Check sheet for the modelled part. Datum: model origin and axes. Units: mm. A direction names the side the tool comes from. Round coordinates to 2 decimals unless told otherwise and drop trailing zeros. Write each loop counter-clockwise with the first axis right and the second up, starting at its lowest first coordinate (ties: lowest second). Pieces come first, ordered by that corner, then holes. Notation, with made-up numbers: (-8.75, -2.75) -> (47.25, -2.75) arc R21 ccw to (47.25, 14.25) -> close; hole circle Ø11 at (-6, 23.25). An arc over 180 degrees is marked (long way). Put each result on its own line as item: value. Start each with the question number.
from build123d import *

# Parameters (mm, degrees)
SKETCH1_W              = 273.05
SKETCH1_H              = 139.7
BOSS_EXTRUDE1_DEPTH    = 5.588
SKETCH2_W              = 273.05
SKETCH2_H              = 139.7
SKETCH2_W_2            = 261.874
SKETCH2_H_2            = 128.524
BOSS_EXTRUDE2_DEPTH    = 298.45
SKETCH3_W              = 6.35
SKETCH3_H              = 16.933333333
SKETCH3_H_2            = 16.933333334
DOOR_SLOT_DEPTH        = 12.7
DOOR_GUIDE_HOLES_REACH = 361.255
SKETCH4_W              = 6.35
SKETCH4_H              = 15.875
LEVER_HOLES_W          = 9.652
LEVER_HOLES_H          = 6.35
LEVER_HOLES_W_2        = 6.35
CUT_EXTRUDE1_DEPTH     = 362.378293578
CUT_EXTRUDE3_REACH     = 416.577
SKETCH8_R              = 3.175
SKETCH16_W             = 327.238778096
SKETCH16_H             = 314.471565403
CUT_EXTRUDE10_DEPTH    = 362.378293578
LEFT_RIGHT_W           = 6.35
LEFT_RIGHT_H           = 5.588
LEFT_RIGHT_W_2         = 12.7
LEFT_RIGHT_H_2         = 12.66825
CUT_EXTRUDE11_DEPTH    = 415.577411883
SKETCH17_R             = 1.5
SKETCH17_W             = 23
SKETCH17_H             = 17.61800007
CUT_EXTRUDE12_DEPTH    = 313.00857951
CUT_EXTRUDE13_DEPTH    = 313.00857951


with BuildPart() as part:
    # Sketch1 → Boss-Extrude1 (new body)
    with BuildSketch(Plane(origin=(0, 0, 0), x_dir=(1, 0, 0), z_dir=(0, 1, 0))):
        Rectangle(SKETCH1_W, SKETCH1_H)
    extrude(amount=BOSS_EXTRUDE1_DEPTH)

    # Sketch2 → Boss-Extrude2 (add)
    with BuildSketch(Plane(origin=(0, 5.588, 0), x_dir=(1, 0, 0), z_dir=(0, 1, 0))):
        Rectangle(SKETCH2_W, SKETCH2_H)
        Rectangle(SKETCH2_W_2, SKETCH2_H_2, mode=Mode.SUBTRACT)
    extrude(amount=BOSS_EXTRUDE2_DEPTH)

    # Sketch3 → Door Slot (cut)
    with BuildSketch(Plane.XY.offset(69.85)):
        with BuildLine():
            Line((-29.337, 282.448), (-29.337, 5.588))
            Line((-29.337, 5.588), (-22.733, 5.588))
            Line((-22.733, 5.588), (-22.733, 291.592))
            Line((-22.733, 291.592), (-42.291, 291.592))
            Line((-42.291, 291.592), (-42.291, 284.988))
            Line((-42.291, 284.988), (-31.877, 284.988))
            ThreePointArc((-31.877, 284.988), (-30.080948776, 284.244051224), (-29.337, 282.448))
        make_face()
        with Locations((-13.208, 80.433333334)):
            Rectangle(SKETCH3_W, SKETCH3_H)
        with Locations((-13.208, 50.8)):
            Rectangle(SKETCH3_W, SKETCH3_H_2)
        with Locations((-13.208, 21.166666667)):
            Rectangle(SKETCH3_W, SKETCH3_H)
    extrude(amount=-DOOR_SLOT_DEPTH, mode=Mode.SUBTRACT)

    # Sketch4 → Door Guide Holes (cut, up to next)
    with BuildSketch(Plane.XY.offset(-64.262), mode=Mode.PRIVATE) as door_guide_holes_sk1:
        with Locations((-45.466, 283.4005)):
            Rectangle(SKETCH4_W, SKETCH4_H)
    door_guide_holes_tool1 = extrude(door_guide_holes_sk1.sketch, amount=-DOOR_GUIDE_HOLES_REACH, mode=Mode.PRIVATE) & part.part
    # Sketch4 → Door Guide Holes (cut, up to next)
    with BuildSketch(Plane.XY.offset(-64.262), mode=Mode.PRIVATE) as door_guide_holes_sk2:
        with Locations((-45.466, 254.8255)):
            Rectangle(SKETCH4_W, SKETCH4_H)
    door_guide_holes_tool2 = extrude(door_guide_holes_sk2.sketch, amount=-DOOR_GUIDE_HOLES_REACH, mode=Mode.PRIVATE) & part.part
    # Sketch4 → Door Guide Holes (cut, up to next)
    with BuildSketch(Plane.XY.offset(-64.262), mode=Mode.PRIVATE) as door_guide_holes_sk3:
        with Locations((-45.466, 226.2505)):
            Rectangle(SKETCH4_W, SKETCH4_H)
    door_guide_holes_tool3 = extrude(door_guide_holes_sk3.sketch, amount=-DOOR_GUIDE_HOLES_REACH, mode=Mode.PRIVATE) & part.part
    # Sketch4 → Door Guide Holes (cut, up to next)
    with BuildSketch(Plane.XY.offset(-64.262), mode=Mode.PRIVATE) as door_guide_holes_sk4:
        with Locations((-45.466, 197.6755)):
            Rectangle(SKETCH4_W, SKETCH4_H)
    door_guide_holes_tool4 = extrude(door_guide_holes_sk4.sketch, amount=-DOOR_GUIDE_HOLES_REACH, mode=Mode.PRIVATE) & part.part
    # Sketch4 → Door Guide Holes (cut, up to next)
    with BuildSketch(Plane.XY.offset(-64.262), mode=Mode.PRIVATE) as door_guide_holes_sk5:
        with Locations((-45.466, 169.1005)):
            Rectangle(SKETCH4_W, SKETCH4_H)
    door_guide_holes_tool5 = extrude(door_guide_holes_sk5.sketch, amount=-DOOR_GUIDE_HOLES_REACH, mode=Mode.PRIVATE) & part.part
    # Sketch4 → Door Guide Holes (cut, up to next)
    with BuildSketch(Plane.XY.offset(-64.262), mode=Mode.PRIVATE) as door_guide_holes_sk6:
        with Locations((-45.466, 140.5255)):
            Rectangle(SKETCH4_W, SKETCH4_H)
    door_guide_holes_tool6 = extrude(door_guide_holes_sk6.sketch, amount=-DOOR_GUIDE_HOLES_REACH, mode=Mode.PRIVATE) & part.part
    # Sketch4 → Door Guide Holes (cut, up to next)
    with BuildSketch(Plane.XY.offset(-64.262), mode=Mode.PRIVATE) as door_guide_holes_sk7:
        with Locations((-45.466, 111.9505)):
            Rectangle(SKETCH4_W, SKETCH4_H)
    door_guide_holes_tool7 = extrude(door_guide_holes_sk7.sketch, amount=-DOOR_GUIDE_HOLES_REACH, mode=Mode.PRIVATE) & part.part
    # Sketch4 → Door Guide Holes (cut, up to next)
    with BuildSketch(Plane.XY.offset(-64.262), mode=Mode.PRIVATE) as door_guide_holes_sk8:
        with Locations((-45.466, 83.3755)):
            Rectangle(SKETCH4_W, SKETCH4_H)
    door_guide_holes_tool8 = extrude(door_guide_holes_sk8.sketch, amount=-DOOR_GUIDE_HOLES_REACH, mode=Mode.PRIVATE) & part.part
    # Sketch4 → Door Guide Holes (cut, up to next)
    with BuildSketch(Plane.XY.offset(-64.262), mode=Mode.PRIVATE) as door_guide_holes_sk9:
        with Locations((-45.466, 54.8005)):
            Rectangle(SKETCH4_W, SKETCH4_H)
    door_guide_holes_tool9 = extrude(door_guide_holes_sk9.sketch, amount=-DOOR_GUIDE_HOLES_REACH, mode=Mode.PRIVATE) & part.part
    # Sketch4 → Door Guide Holes (cut, up to next)
    with BuildSketch(Plane.XY.offset(-64.262), mode=Mode.PRIVATE) as door_guide_holes_sk10:
        with Locations((-45.466, 26.2255)):
            Rectangle(SKETCH4_W, SKETCH4_H)
    door_guide_holes_tool10 = extrude(door_guide_holes_sk10.sketch, amount=-DOOR_GUIDE_HOLES_REACH, mode=Mode.PRIVATE) & part.part
    door_guide_holes_1 = door_guide_holes_tool1.solids().sort_by_distance((-45.466, 283.4005, -64.262))[0]
    add(door_guide_holes_1, mode=Mode.SUBTRACT)
    door_guide_holes_2 = door_guide_holes_tool2.solids().sort_by_distance((-45.466, 254.8255, -64.262))[0]
    add(door_guide_holes_2, mode=Mode.SUBTRACT)
    door_guide_holes_3 = door_guide_holes_tool3.solids().sort_by_distance((-45.466, 226.2505, -64.262))[0]
    add(door_guide_holes_3, mode=Mode.SUBTRACT)
    door_guide_holes_4 = door_guide_holes_tool4.solids().sort_by_distance((-45.466, 197.6755, -64.262))[0]
    add(door_guide_holes_4, mode=Mode.SUBTRACT)
    door_guide_holes_5 = door_guide_holes_tool5.solids().sort_by_distance((-45.466, 169.1005, -64.262))[0]
    add(door_guide_holes_5, mode=Mode.SUBTRACT)
    door_guide_holes_6 = door_guide_holes_tool6.solids().sort_by_distance((-45.466, 140.5255, -64.262))[0]
    add(door_guide_holes_6, mode=Mode.SUBTRACT)
    door_guide_holes_7 = door_guide_holes_tool7.solids().sort_by_distance((-45.466, 111.9505, -64.262))[0]
    add(door_guide_holes_7, mode=Mode.SUBTRACT)
    door_guide_holes_8 = door_guide_holes_tool8.solids().sort_by_distance((-45.466, 83.3755, -64.262))[0]
    add(door_guide_holes_8, mode=Mode.SUBTRACT)
    door_guide_holes_9 = door_guide_holes_tool9.solids().sort_by_distance((-45.466, 54.8005, -64.262))[0]
    add(door_guide_holes_9, mode=Mode.SUBTRACT)
    door_guide_holes_10 = door_guide_holes_tool10.solids().sort_by_distance((-45.466, 26.2255, -64.262))[0]
    add(door_guide_holes_10, mode=Mode.SUBTRACT)
    door_guide_holes = door_guide_holes_1 + door_guide_holes_2 + door_guide_holes_3 + door_guide_holes_4 + door_guide_holes_5 + door_guide_holes_6 + door_guide_holes_7 + door_guide_holes_8 + door_guide_holes_9 + door_guide_holes_10  # Door Guide Holes as one shape, for the pattern or mirror that repeats it

    # Mirror1: Door Guide Holes across plane
    add(door_guide_holes.mirror(Plane.ZY.offset(32.512)), mode=Mode.SUBTRACT)

    # Lever Holes → Cut-Extrude1 (cut, through all)
    with BuildSketch(Plane.XY.offset(69.85)):
        with Locations((54.102, 28.575)):
            Rectangle(LEVER_HOLES_W, LEVER_HOLES_H)
        with Locations((39.3065, 15.875)):
            Rectangle(LEVER_HOLES_W_2, LEVER_HOLES_H)
        with Locations((68.8975, 15.875)):
            Rectangle(LEVER_HOLES_W_2, LEVER_HOLES_H)
    extrude(amount=-CUT_EXTRUDE1_DEPTH, mode=Mode.SUBTRACT)

    # Sketch8 → Cut-Extrude3 (cut, up to next)
    with BuildSketch(Plane.ZY.offset(136.525), mode=Mode.PRIVATE) as cut_extrude3_sk1:
        with Locations((0, 19.05)):
            Circle(SKETCH8_R)
    cut_extrude3_tool1 = extrude(cut_extrude3_sk1.sketch, amount=-CUT_EXTRUDE3_REACH, mode=Mode.PRIVATE) & part.part
    add(cut_extrude3_tool1.solids().sort_by_distance((-136.525, 19.05, 0))[0], mode=Mode.SUBTRACT)

    # Sketch16 → Cut-Extrude10 (cut, through all)
    with BuildSketch(Plane.XY.offset(69.85)):
        with Locations((-32.682389048, 146.802217299)):
            Rectangle(SKETCH16_W, SKETCH16_H)
    extrude(amount=-CUT_EXTRUDE10_DEPTH, mode=Mode.SUBTRACT)

    # Left/Right → Cut-Extrude11 (cut, through all)
    with BuildSketch(Plane.ZY.offset(136.525)):
        with Locations((60.325, 2.794)):
            Rectangle(LEFT_RIGHT_W, LEFT_RIGHT_H)
        with Locations((38.1, 2.794)):
            Rectangle(LEFT_RIGHT_W_2, LEFT_RIGHT_H)
        with Locations((66.675, 19.002375)):
            Rectangle(LEFT_RIGHT_W, LEFT_RIGHT_H_2)
        with Locations((12.7, 2.794)):
            Rectangle(LEFT_RIGHT_W_2, LEFT_RIGHT_H)
        with Locations((66.675, 44.338875)):
            Rectangle(LEFT_RIGHT_W, LEFT_RIGHT_H_2)
        with Locations((-12.7, 2.794)):
            Rectangle(LEFT_RIGHT_W_2, LEFT_RIGHT_H)
        with Locations((66.675, 69.675375)):
            Rectangle(LEFT_RIGHT_W, LEFT_RIGHT_H_2)
        with Locations((-38.1, 2.794)):
            Rectangle(LEFT_RIGHT_W_2, LEFT_RIGHT_H)
        with Locations((66.675, 95.011875)):
            Rectangle(LEFT_RIGHT_W, LEFT_RIGHT_H_2)
        with Locations((-60.325, 2.794)):
            Rectangle(LEFT_RIGHT_W, LEFT_RIGHT_H)
        with Locations((66.675, 120.348375)):
            Rectangle(LEFT_RIGHT_W, LEFT_RIGHT_H_2)
        with Locations((-66.675, 19.002375)):
            Rectangle(LEFT_RIGHT_W, LEFT_RIGHT_H_2)
        with Locations((66.675, 145.684875)):
            Rectangle(LEFT_RIGHT_W, LEFT_RIGHT_H_2)
        with Locations((-66.675, 44.338875)):
            Rectangle(LEFT_RIGHT_W, LEFT_RIGHT_H_2)
        with Locations((66.675, 171.021375)):
            Rectangle(LEFT_RIGHT_W, LEFT_RIGHT_H_2)
        with Locations((-66.675, 69.675375)):
            Rectangle(LEFT_RIGHT_W, LEFT_RIGHT_H_2)
        with Locations((66.675, 196.357875)):
            Rectangle(LEFT_RIGHT_W, LEFT_RIGHT_H_2)
        with Locations((-66.675, 95.011875)):
            Rectangle(LEFT_RIGHT_W, LEFT_RIGHT_H_2)
        with Locations((66.675, 221.694375)):
            Rectangle(LEFT_RIGHT_W, LEFT_RIGHT_H_2)
        with Locations((-66.675, 120.348375)):
            Rectangle(LEFT_RIGHT_W, LEFT_RIGHT_H_2)
        with Locations((66.675, 247.030875)):
            Rectangle(LEFT_RIGHT_W, LEFT_RIGHT_H_2)
        with Locations((-66.675, 145.684875)):
            Rectangle(LEFT_RIGHT_W, LEFT_RIGHT_H_2)
        with Locations((66.675, 272.367375)):
            Rectangle(LEFT_RIGHT_W, LEFT_RIGHT_H_2)
        with Locations((-66.675, 171.021375)):
            Rectangle(LEFT_RIGHT_W, LEFT_RIGHT_H_2)
        with Locations((66.675, 297.703875)):
            Rectangle(LEFT_RIGHT_W, LEFT_RIGHT_H_2)
        with Locations((-66.675, 196.357875)):
            Rectangle(LEFT_RIGHT_W, LEFT_RIGHT_H_2)
        with Locations((-66.675, 221.694375)):
            Rectangle(LEFT_RIGHT_W, LEFT_RIGHT_H_2)
        with Locations((-66.675, 247.030875)):
            Rectangle(LEFT_RIGHT_W, LEFT_RIGHT_H_2)
        with Locations((-66.675, 272.367375)):
            Rectangle(LEFT_RIGHT_W, LEFT_RIGHT_H_2)
        with Locations((-66.675, 297.703875)):
            Rectangle(LEFT_RIGHT_W, LEFT_RIGHT_H_2)
    extrude(amount=-CUT_EXTRUDE11_DEPTH, mode=Mode.SUBTRACT)

    # Sketch17 → Cut-Extrude12 (cut, through all)
    with BuildSketch(Plane(origin=(136.525, 0, 0), x_dir=(0, 0, -1), z_dir=(1, 0, 0))):
        with Locations((-8, 62.088)):
            Circle(SKETCH17_R)
        with Locations((8, 62.088)):
            Circle(SKETCH17_R)
        with Locations((-50.8, 159.894)):
            Circle(SKETCH17_R)
        with Locations((-50.8, 144.144)):
            Circle(SKETCH17_R)
        with Locations(Location((50.8, 144.144, 0), (0, 0, 180))):
            Circle(SKETCH17_R)
        with Locations(Location((50.8, 159.894, 0), (0, 0, 180))):
            Circle(SKETCH17_R)
        with Locations((0, 22.779000035)):
            Rectangle(SKETCH17_W, SKETCH17_H)
    extrude(amount=-CUT_EXTRUDE12_DEPTH, mode=Mode.SUBTRACT)

    # Sketch18 → Cut-Extrude13 (cut, through all)
    with BuildSketch(Plane(origin=(136.525, 0, 0), x_dir=(0, 0, -1), z_dir=(1, 0, 0))):
        Polygon((-69.85, 304.038), (-69.85, 0), (-25.4, 0), (-25.4, 5.588), (-30.988, 5.588), (-30.988, 18.288), (-25.4, 18.288), (-25.4, 30.48), (-30.988, 30.48), (-30.988, 43.18), (-25.4, 43.18), (-25.4, 101.346), (25.4, 101.346), (25.4, 43.18), (30.988, 43.18), (30.988, 30.48), (25.4, 30.48), (25.4, 18.288), (30.988, 18.288), (30.988, 5.588), (25.4, 5.588), (25.4, 0), (69.85, 0), (69.85, 304.038), align=None)
    extrude(amount=-CUT_EXTRUDE13_DEPTH, mode=Mode.SUBTRACT)


solid = part.part
1. Gauge pin test, flat ends, axial feed: P1, Ø3, axis at x = 132.5, z = -27.5, coming from the +Y side; P2, Ø3, axis at x = 132.5, y = 1.5, coming from the +Z side; P3, Ø3, axis at x = 134, z = 9.5, coming from the -Y side; P4, Ø2.5, axis at y = 62.088, z = 8, coming from the +X side. Record the tip position at first contact, or that the pin passes through.
2. Section check C-C, the plane y = 48.5. Enter the section's corners in (x, z) (3 decimals), then the cut area to 3 significant figures.
3. Section check A-A, the plane z = 10.5. Enter the section's corners in (x, y) (3 decimals), then the cut area to 3 significant figures.
4. Material ranges on L1, parallel to Y at x = 133.55, z = 8; L2, parallel to Z at x = 133.1, y = 5; L3, parallel to Y at x = 134.5, z = -10, recorded low to high. Write a range as [from, to].
5. Access from +Z, -Z, +X, -X, +Y, -Y to the whole of each face (thin tool, end or side, straight path). Record for faces 1 (the flat face through (134, 30.48, 28)), 2 (the flat face through (134, 3, 6.35)), 3 (the flat face through (134, 31.588, 0)).
6. Draft check along Y on faces 4 (the flat face through (134, 5.588, 13)), 5 (the flat face through (134, 13.97, 0)), 6 (the flat face through (134, 12, -30.988)). Enter one of: released by +Y, released by -Y, zero draft, split by the parting line, or undercut.
7. Section check B-B, the plane x = 132.85. Give the number of separate pieces and of enclosed holes in the cut face, then the cut area to 3 significant figures.
Reply:
1. P1: stops at y = 43.18
1. P2: stops at z = 25.4
1. P3: stops at y = 5.59
1. P4: passes through
2. outline: (130.937, -25.4) -> (136.525, -25.4) -> (136.525, 25.4) -> (130.937, 25.4) -> close
2. area: 284 mm2
3. outline: (130.937, 5.588) -> (136.525, 5.588) -> (136.525, 13.97) -> (130.937, 13.97) -> close; (130.937, 31.588) -> (136.525, 31.588) -> (136.525, 101.346) -> (130.937, 101.346) -> close
3. area: 437 mm2
4. L1: y = [5.59, 13.97], [31.59, 60.59], [63.59, 101.35]
4. L2: z = [-25.4, -19.05], [-6.35, 6.35], [19.05, 25.4]
4. L3: y = [5.59, 13.97], [31.59, 101.35]
5. face 1: +Z, +X, -X
5. face 2: +X, -X, -Y
5. face 3: +X, -X
6. face 4: released by -Y
6. face 5: undercut
6. face 6: zero draft
7. separate pieces: 1
7. enclosed holes: 3
7. area: 4,870 mm2
